from build123d import *

# Parameters (mm, degrees)
F0_R     = 1.6
F1_DEPTH = 4
F0_W     = 14
F0_H     = 4
F2_DEPTH = 25.4
F3_R     = 1.6
F4_DEPTH = 4
F5_R     = 3.99999


# Not quite as in the source:
# - a fillet or chamfer is up to 0.001 mm smaller than in the source, because OpenCascade refuses the exact size


with BuildPart() as f1:
    # F0 (on Top) → F1 (new body)
    with BuildSketch(Plane.XY):
        Polygon((7, 12.7), (-7, 12.7), (-7, -8.7), (7, -8.7), (7, -0.5), (15.1, -0.5), (15.1, 12.7), align=None)
        with Locations((0, -2.1)):
            Circle(F0_R, mode=Mode.SUBTRACT)
        with Locations((0, 6.1)):
            Circle(F0_R, mode=Mode.SUBTRACT)
        with Locations((9.5, 6.1)):
            Circle(F0_R, mode=Mode.SUBTRACT)
    extrude(amount=-F1_DEPTH)

    # F0 (on Top) → F2 (join)
    with BuildSketch(Plane.XY):
        with Locations((0, -10.7)):
            Rectangle(F0_W, F0_H)
    extrude(amount=-F2_DEPTH)

    # F3 (on face) → F4 (cut, through all)
    with BuildSketch(Plane(origin=(0, -8.7, 0), x_dir=(-1, 0, 0), z_dir=(0, 1, 0))):
        with Locations((0, -10.6)):
            Circle(F3_R)
        with Locations((0, -18.8)):
            Circle(F3_R)
    extrude(amount=-F4_DEPTH, mode=Mode.SUBTRACT)

    # F5 (radius 4 in the source; OpenCascade refuses exactly that, so slightly less here)
    f5_edges = [f1.edges().sort_by_distance(p)[0] for p in [
        (-7, -8.7, -14.7),
        (0, -8.7, -25.4),
        (7, -8.7, -14.7),
        (-7, 2, -4),
        (7, -4.6, -4),
        (11.05, -0.5, -4),
    ]]
    fillet(f5_edges, radius=F5_R)


solid = f1.part
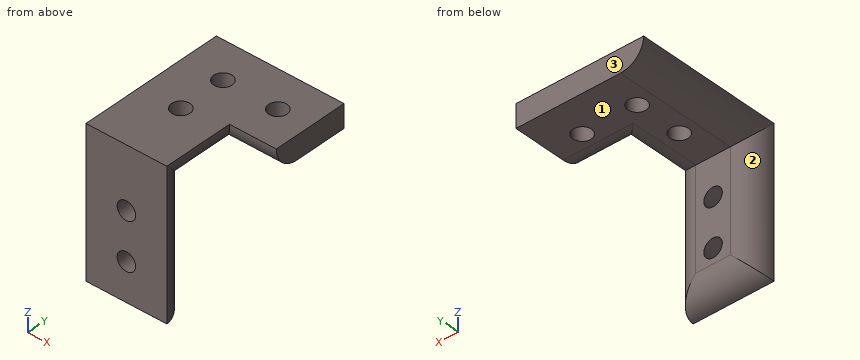
Verification items for the finished model (mm, model axes). Face numbers are marked on the shaded views. A direction names the side the tool comes from. Coordinates: 2 decimals unless noted, no trailing zeros. One line per item, written item: value. Start each with the question number.
Q1. Thickness scan on L1, parallel to Y at x = 0, z = -2; L2, parallel to Z at x = 8.5, y = 9.75; L3, parallel to Z at x = 0, y = -11.8. Record the ranges inside material, lowest first. Write a range as from..to.
Q2. Access from +Z, -Z, +X, -X, +Y, -Y to the whole of each face (thin tool, end or side, straight path). Record for the marked faces 1, 2 and 3.
Q3. Cross-section at A-A on y = 6.1. State how many separate pieces and enclosed holes the cut face has, and give its area (3 significant figures).
Q4. Go/stop test with flat-tipped pins: P1, Ø4, axis at x = 3, z = -7.5, coming from the +Y side; P2, Ø5.5, axis at x = 6.5, y = 2, coming from the -Z side; P3, Ø13.5, axis at y = -4.5, z = -14, coming from the +X side. Record where each tip stops, or that it passes through.
Checked values:
1. L1: y = -12.7..-3.7, -0.5..4.5, 7.7..12.7
1. L2: z = -4..0
1. L3: z = -25.3..-20.4, -17.2..-12.2, -9..0
2. face 1: -Z, +X, -X, +Y
2. face 2: -Z, -X, +Y
2. face 3: +Z, -Z, +X, -X, +Y
3. separate pieces: 3
3. enclosed holes: 0
3. area: 59.4 mm²
4. P1: stops at y = -8.7
4. P2: stops at z = -4
4. P3: stops at x = 6.73
